Source: CAD feature listing. Evaluate the final solid. Frame: model axes, mm. A direction names the side the tool comes from. Give positions to 0.01 mm unless a question says otherwise; leave off trailing zeros. Loops run counter-clockwise (first coordinate to the right, second up) from the corner with the lowest first, then second, coordinate; pieces in that order, holes last.
Autodesk Inventor part; units mm, degrees
ref_plane "YZ Plane" through (0, 0, 0) normal (1, 0, 0) x (0, 1, 0)
ref_plane "XZ Plane" through (0, 0, 0) normal (0, 1, 0) x (-1, 0, 0)
ref_plane "XY Plane" through (0, 0, 0) normal (0, 0, 1) x (1, 0, 0)
sketch "Boceto1" plane through (0, 0, 0) normal (0, 1, 0) x (-1, 0, 0)
  circle A0 centre (0, 0) radius 12.446
  dimension "d0" = 24.892
extrude "Extrusión1" add sketch "Boceto1" along normal blind 48.006
sketch "Boceto2" plane through (0, 0, 0) normal (0, -1, 0) x (1, 0, 0)
  arc A0 (-1.3229, 1.5) -> (1.3229, 1.5) centre (0, 0) ccw
  line L0 (-1.3229, 1.5) -> (1.3229, 1.5)
  dimension "d3" = 4
  dimension "d4" = 1.5
extrude "Extrusión2" add sketch "Boceto2" along normal blind 8.001
sketch "Boceto3" plane through (0, 0, 0) normal (0, -1, 0) x (1, 0, 0)
  arc A0 (-1.3229, 1.5) -> (1.3229, 1.5) centre (0, 0) ccw
  point P0 (0, 8.5)
  point P1 (-8.5, 0)
  point P2 (0, -8.5)
  point P3 (8.5, 0)
  dimension "d7" = 8.5
  dimension "d10" = 360
hole "Hole1" at (0, 0, 8.5) at (-8.5, 0, 0) at (0, 0, -8.5) at (8.5, 0, 0) direction (0, 1, 0) diameter 2.459 depth 6 tip angle 118
properties part number "Motor" material "Aluminio-6061"
(1) First-contact query: pin 1 (2 mm diameter, centred on x = 8.5, z = 0, fed in from -Y); pin 2 (1.5 mm diameter, centred on x = -8.5, z = 0, fed in from -Y); pin 3 (1.5 mm diameter, centred on y = 22.5, z = 3, fed in from -X). Flat tips, straight axial feed; report the tip coordinate or a pass-through.
A:
pin 1: stops at y = 6.14
pin 2: stops at y = 6.29
pin 3: stops at x = -12.24
(2) Ray query, line 1 along Z through (x, y) = (0, 4.65); line 2 along Y through (x, z) = (2.75, 4.5); line 3 along Z through (x, y) = (0.5, 8). Return the intervals inside material, ascending.
A:
line 1: z = -12.45 to -9.73, -7.27 to 7.27, 9.73 to 12.45
line 2: y = 0 to 48.01
line 3: z = -12.44 to 12.44
(3) Section D-D, the plane y = 28. Return the cut outline in (x, z).
A:
outline: circle Ø24.89 at (0, 0)
(4) Section C-C, the plane x = -5.75. Return the cut outline in (y, z), then the cut area to 3 significant figures.
A:
outline: (0, -11.04) - (48.01, -11.04) - (48.01, 11.04) - (0, 11.04) - close
area: 1,060 mm2
(5) Section B-B, the plane z = 5.75. Return the cut outline in (x, y), then the cut area to 3 significant figures.
A:
outline: (-11.04, 0) - (11.04, 0) - (11.04, 48.01) - (-11.04, 48.01) - close
area: 1,060 mm2
(6) Reachability of faces 4 (the cylindrical face through (2.7, 23.67, 12.15)), 5 (the flat face through (0, -4, 1.5)), 6 (the cylindrical face through (-0.369, 3.042, -9.673)) from +Z, -Z, +X, -X, +Y, -Y: full face, straight path, thin tool, end or side. Return the list, or none.
A:
face 4: +Y, -Y
face 5: +Z, +X, -X, -Y
face 6: -Y
(7) Section A-A, the plane y = 4.5. Return the cut outline in (x, z).
A:
outline: circle Ø24.89 at (0, 0); hole circle Ø2.46 at (-8.5, 0); hole circle Ø2.46 at (0, -8.5); hole circle Ø2.46 at (0, 8.5); hole circle Ø2.46 at (8.5, 0)
(8) Mould query, pull axis Z, two halves, no side actions, for faces 1 (the cylindrical face through (0, -4, -2)), 2 (the flat face through (0, -8.001, 0)), 3 (the cylindrical face through (-7.3, 3.04, 0.27)). Classes: pulls with the +Z half, pulls with the -Z half, needs draft (parallel to the pull), parting line crosses it, or undercut.
A:
face 1: parting line crosses it
face 2: needs draft
face 3: undercut
